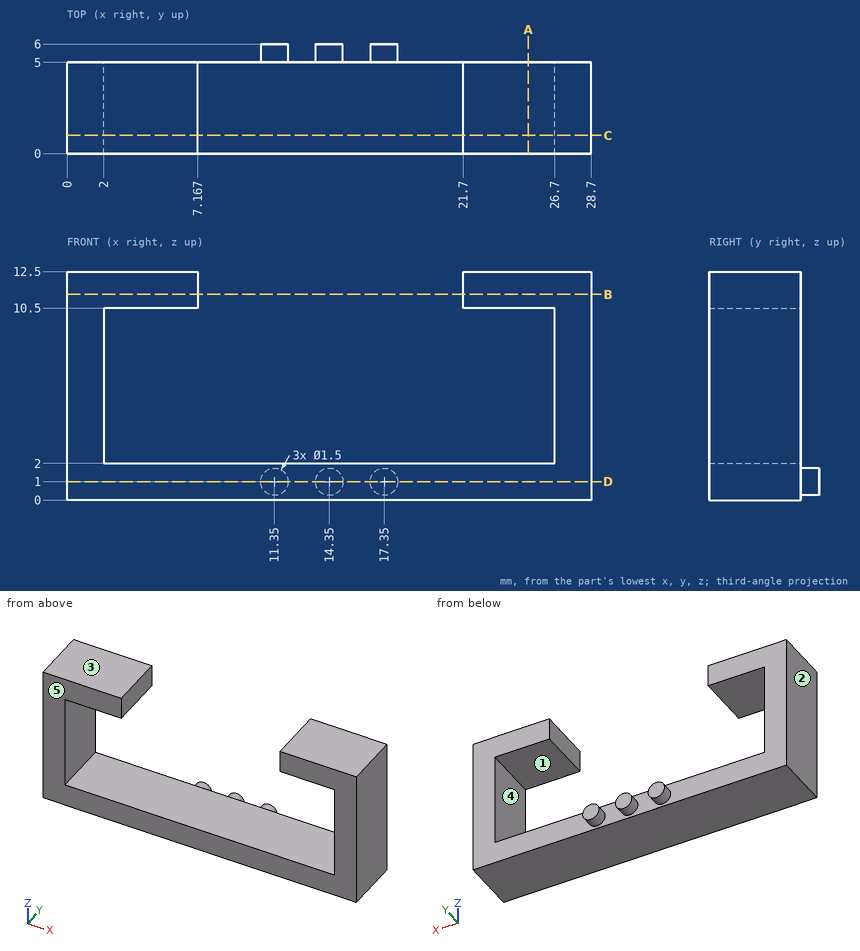
Can you work these out from the drawing? Everything is in mm from the part's minimum corner. A direction names the side the tool comes from. Coordinates: 2 decimals unless noted, no trailing zeros. Loops run counter-clockwise (first coordinate to the right, second up) from the corner with the lowest first, then second, coordinate; pieces in that order, holes last. Notation, with made-up numbers: M -35,43.5 L -22,43.5 A18 cw -22,47.5 Z; hole C 13.5,61 d7. An arc over 180 degrees is marked long. Put each result on its own line as item: value. Start each with the question number.
(1) I need wall thicknesses on line 1 (X direction, y = 1.05, z = 4.75); line 2 (Z direction, x = 24.25, y = 2.65); line 3 (Y direction, x = 26.75, z = 8.5). Which ranges of each line are inside material? Lowest first, please. Write a range as from..to.
(2) Suppose I cut it at B-B on z = 11.25. Please give me the cut outline in (x, y), then the cut area to 3 significant figures.
(3) Suppose I cut it at C-C on y = 1. Please give me the cut outline in (x, z), then the cut area to 3 significant figures.
(4) Suppose I cut it at D-D on z = 1. Please give me the cut outline in (x, y).
(5) For the marked faces 4 and 5, which set-ups out of +Z, -Z, +X, -X, +Y, -Y let a thin tool reach every point of the face, with its end or its side?
(6) Suppose I cut it at A-A on x = 25.25. Please give me the cut outline in (y, z).
(7) Thinking about a two-plate mould opening in X: for the marked faces 1, 2 and 3, which applies, pulls with the +X half, pulls with the -X half, needs draft (parallel to the pull), parting line crosses it, or undercut?
Solutions:
1. line 1: x = 0..2, 26.7..28.7
1. line 2: z = 0..2, 10.5..12.5
1. line 3: y = 0..5
2. outline: M 0,0 L 7.17,0 L 7.17,5 L 0,5 Z; M 21.7,0 L 28.7,0 L 28.7,5 L 21.7,5 Z
2. area: 70.8 mm2
3. outline: M 0,0 L 28.7,0 L 28.7,12.5 L 21.7,12.5 L 21.7,10.5 L 26.7,10.5 L 26.7,2 L 2,2 L 2,10.5 L 7.17,10.5 L 7.17,12.5 L 0,12.5 Z
3. area: 120 mm2
4. outline: M 0,0 L 28.7,0 L 28.7,5 L 18.1,5 L 18.1,6 L 16.6,6 L 16.6,5 L 15.1,5 L 15.1,6 L 13.6,6 L 13.6,5 L 12.1,5 L 12.1,6 L 10.6,6 L 10.6,5 L 0,5 Z
5. face 4: +Y, -Y
5. face 5: +Z, -Z, +X, -X, -Y
6. outline: M 0,0 L 5,0 L 5,2 L 0,2 Z; M 0,10.5 L 5,10.5 L 5,12.5 L 0,12.5 Z
7. face 1: undercut
7. face 2: pulls with the -X half
7. face 3: needs draft
